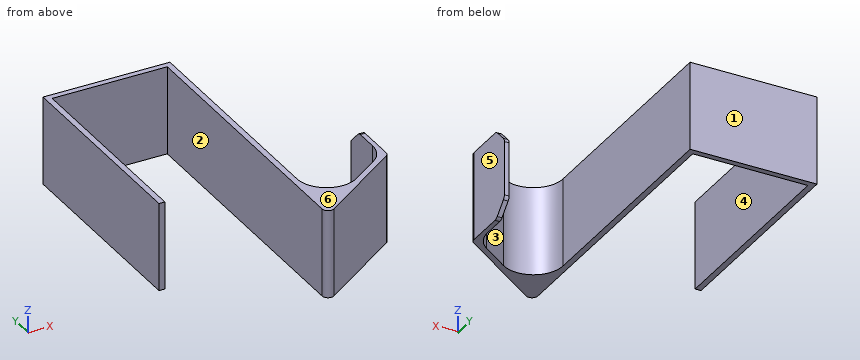
from build123d import *

# Parameters (mm, degrees)
BOSS_EXTRU_1_DEPTH = 30
CONG_1_R           = 10
CHANFREIN1_SIZE    = 5
CONG_2_R           = 2


with BuildPart() as part:
    # Esquisse1 → Boss.-Extru.1 (new body)
    with BuildSketch(Plane.XY):
        Polygon((-19.55, 43.689057372), (-19.55, 113.689057372), (19.55, 113.689057372), (19.55, 13.689057372), (52.316081772, 36.632114826), (52.316081772, 56.632114826), (50.716081772, 56.632114826), (50.716081772, 37.953331942), (21.55, 17.531021626), (21.55, 115.689057372), (-21.55, 115.689057372), (-21.55, 43.689057372), align=None)
    extrude(amount=BOSS_EXTRU_1_DEPTH)

    # Congé1
    cong_1_edges = [part.edges().sort_by_distance(p)[0] for p in [
        (21.55, 17.531021626, 15),
        (50.716081772, 37.953331942, 15),
    ]]
    fillet(cong_1_edges, radius=CONG_1_R)

    # Chanfrein1
    chanfrein1_edges = [part.edges().sort_by_distance(p)[0] for p in [
        (51.516081772, 56.632114826, 0),
        (51.516081772, 56.632114826, 30),
    ]]
    chamfer(chanfrein1_edges, length=CHANFREIN1_SIZE)

    # Congé2
    cong_2_edges = [part.edges().sort_by_distance(p)[0] for p in [
        (52.316081772, 36.632114826, 15),
        (19.55, 13.689057372, 15),
        (51.516081772, 56.632114826, 25),
        (51.516081772, 56.632114826, 5),
        (51.516081772, 51.632114826, 0),
        (51.516081772, 51.632114826, 30),
    ]]
    fillet(cong_2_edges, radius=CONG_2_R)


solid = part.part
The listing builds one solid part. Answer for the finished solid, in the listing's coordinates (mm). Face numbers are marked on the shaded views. A direction names the side the tool comes from. Coordinates: 2 decimals unless noted, no trailing zeros. Loops run counter-clockwise (first coordinate to the right, second up) from the corner with the lowest first, then second, coordinate; pieces in that order, holes last. Notation, with made-up numbers: (64.5, 55.5) -> (72.5, 55.5) arc R27 cw to (72.5, 94.5) -> close; hole circle Ø11 at (27.25, 35). An arc over 180 degrees is marked (long way). Answer in a Markdown table with one row per item. Add a question column.
1. The part is cut by section B-B, the plane z = 9. Write down the section's boundary in (x, y), then the cut area to 4 significant figures.
2. Determine the mould class of the marked faces 4, 5 and 6 for opening direction X: +X half, -X half, draft (parallel to the pull), parting line (faces both ways), or undercut.
3. The part is cut by section D-D, the plane z = 2.25. Write down the section's boundary in (x, y).
4. For the marked faces 1, 2 and 3, determine the directions among +Z, -Z, +X, -X, +Y, -Y from which every point of the face is accessible in a straight line to the end or side of a thin tool.
5. Consider line 1 (X direction, y = 70, z = 12.5); line 2 (Y direction, x = -8, z = 17). Determine where each line is inside the solid, lowest interval first. Write a range as [from, to].
6. The part is cut by section A-A, the plane y = 64. Write down the section's boundary in (x, z), then the cut area to 3 significant figures.
7. Flat-ended cylindrical pins translate along their axes: P1, Ø1, axis at x = -21, z = 8, coming from the -Y side; P2, Ø1, axis at y = 32, z = 13, coming from the +X side; P3, Ø2, axis at x = 27, z = 19.5, coming from the +Y side; P4, Ø9, axis at y = 58.5, z = 18.5, coming from the +X side. Find the tip coordinate at first contact, or state that the pin passes through.
8. The part is cut by section C-C, the plane x = 9. Write down the section's boundary in (y, z), then the cut area to 3 significant figures.
Answer below:
| question | item | result |
|---|---|---|
| 1 | outline | (-21.55, 43.69) -> (-19.55, 43.69) -> (-19.55, 113.69) -> (19.55, 113.69) -> (19.55, 17.53) arc R2 ccw to (22.7, 15.89) -> (51.46, 36.03) arc R2 ccw to (52.32, 37.67) -> (52.32, 56.63) -> (50.72, 56.63) -> (50.72, 43.16) arc R10 cw to (46.45, 34.97) -> (37.29, 28.55) arc R10 cw to (21.55, 36.74) -> (21.55, 115.69) -> (-21.55, 115.69) -> close |
| 1 | area | 612.5 mm2 |
| 2 | face 4 | undercut |
| 2 | face 5 | +X half |
| 2 | face 6 | draft |
| 3 | outline | (-21.55, 43.69) -> (-19.55, 43.69) -> (-19.55, 113.69) -> (19.55, 113.69) -> (19.55, 17.53) arc R2 ccw to (22.7, 15.89) -> (51.46, 36.03) arc R2 ccw to (52.32, 37.67) -> (52.32, 53.88) -> (50.72, 53.88) -> (50.72, 43.16) arc R10 cw to (46.45, 34.97) -> (37.29, 28.55) arc R10 cw to (21.55, 36.74) -> (21.55, 115.69) -> (-21.55, 115.69) -> close |
| 4 | face 1 | +Z, -Z, +X, -X, +Y |
| 4 | face 2 | +Z, -Z, -Y |
| 4 | face 3 | +Z, -Z, +Y |
| 5 | line 1 | [-21.55, -19.55], [19.55, 21.55] |
| 5 | line 2 | [113.69, 115.69] |
| 6 | outline | (-21.55, 0) -> (-19.55, 0) -> (-19.55, 30) -> (-21.55, 30) -> close; (19.55, 0) -> (21.55, 0) -> (21.55, 30) -> (19.55, 30) -> close |
| 6 | area | 120 mm2 |
| 7 | P1 | y = 43.69 |
| 7 | P2 | x = 46.41 |
| 7 | P3 | y = 28.42 |
| 7 | P4 | x = 52.32 |
| 8 | outline | (113.69, 0) -> (115.69, 0) -> (115.69, 30) -> (113.69, 30) -> close |
| 8 | area | 60.0 mm2 |
